```python
from build123d import *

# Parameters (mm, degrees)
BOSS_EXTRUDE1_DEPTH     = 70
SKETCH2_R               = 2.5
CUT_EXTRUDE1_DEPTH      = 81.774377125
CUT_EXTRUDE2_DEPTH      = 81.774377125
CUT_EXTRUDE2_DEPTH_BACK = 81.774377125
SKETCH3_W               = 52
SKETCH3_H               = 57
SKETCH4_R               = 28.5
BOSS_EXTRUDE2_DEPTH     = 52
SKETCH5_R               = 20
BOSS_EXTRUDE3_DEPTH     = 2.5
SKETCH6_R               = 7
BOSS_EXTRUDE4_DEPTH     = 31.5
CUT_EXTRUDE3_DEPTH      = 5


with BuildPart() as part:
    # Sketch1 → Boss-Extrude1 (new body)
    with BuildSketch(Plane.XY):
        Polygon((-28.5, -25.5), (-25.5, -28.5), (25.5, -28.5), (28.5, -25.5), (28.5, 25.5), (25.5, 28.5), (-25.5, 28.5), (-28.5, 25.5), align=None)
    extrude(amount=BOSS_EXTRUDE1_DEPTH)

    # Sketch2 → Cut-Extrude1 (cut, through all)
    with BuildSketch(Plane(origin=(0, 0, 0), x_dir=(-1, 0, 0), z_dir=(0, 0, -1))):
        with Locations((-23.57, 23.57)):
            Circle(SKETCH2_R)
        with Locations((-23.57, -23.57)):
            Circle(SKETCH2_R)
        with Locations((23.57, -23.57)):
            Circle(SKETCH2_R)
        with Locations((23.57, 23.57)):
            Circle(SKETCH2_R)
    extrude(amount=-CUT_EXTRUDE1_DEPTH, mode=Mode.SUBTRACT)

    # Sketch3 → Cut-Extrude2 (cut, two sides: drawn at the far end of the back side and taken through both)
    with BuildSketch(Plane(origin=(0, 0, 0), x_dir=(0, 0, -1), z_dir=(1, 0, 0)).offset(-CUT_EXTRUDE2_DEPTH_BACK)):
        with Locations((-35, 0)):
            Rectangle(SKETCH3_W, SKETCH3_H)
    extrude(amount=CUT_EXTRUDE2_DEPTH + CUT_EXTRUDE2_DEPTH_BACK, mode=Mode.SUBTRACT)


with BuildPart() as cut_extrude2_piece_1:
    # of the separate pieces the step leaves, piece 1, a body of its own (cut_extrude2_pieces)
    add(part.part.solids().sort_by_distance((-28.5, -25.5, 61))[0])



with BuildPart() as cut_extrude2_piece_2:
    # of the separate pieces the step leaves, piece 2, a body of its own (cut_extrude2_pieces)
    add(part.part.solids().sort_by_distance((-28.5, -25.5, 0))[0])


with BuildPart() as cut_extrude2_piece_1_1:
    add(cut_extrude2_piece_1.part)

    add(cut_extrude2_piece_2.part)  # Boss-Extrude2 merges Cut-Extrude2 piece 2
    # Sketch4 → Boss-Extrude2 (add)
    with BuildSketch(Plane.XY.offset(9)):
        with Locations(Location((0, 0, 0), (0, 0, 180))):
            Circle(SKETCH4_R)
    extrude(amount=BOSS_EXTRUDE2_DEPTH)

    # Sketch5 → Boss-Extrude3 (add)
    with BuildSketch(Plane.XY.offset(70)):
        Circle(SKETCH5_R)
    extrude(amount=BOSS_EXTRUDE3_DEPTH)

    # Sketch6 → Boss-Extrude4 (add)
    with BuildSketch(Plane.XY.offset(72.5)):
        Circle(SKETCH6_R)
    extrude(amount=BOSS_EXTRUDE4_DEPTH)

    # Sketch7 → Cut-Extrude3 (cut)
    with BuildSketch(Plane(origin=(0, 9, 0), x_dir=(1, 0, 0), z_dir=(0, 1, 0))):
        with BuildLine():
            Line((-2.5, -98.25), (-2.5, -78.25))
            ThreePointArc((-2.5, -78.25), (0, -75.75), (2.5, -78.25))
            Line((2.5, -78.25), (2.5, -98.25))
            ThreePointArc((2.5, -98.25), (0, -100.75), (-2.5, -98.25))
        make_face()
    extrude(amount=-CUT_EXTRUDE3_DEPTH, mode=Mode.SUBTRACT)


solid = cut_extrude2_piece_1_1.part
```
The listing builds one solid part. Answer for the finished solid, in the listing's coordinates (mm). A direction names the side the tool comes from. Coordinates: 2 decimals unless noted, no trailing zeros. Write each loop counter-clockwise with the first axis right and the second up, starting at its lowest first coordinate (ties: lowest second). Pieces come first, ordered by that corner, then holes. Notation, with made-up numbers: M -32.5,64.5 L 3.5,64.5 A13 cw 3.5,85.5 Z; hole C -6.75,29.5 d4. An arc over 180 degrees is marked long. Use a Markdown table: item, result. Add a question column.
1. Section D-D (x = 15.5) is taken. Give the vertices of the cut face in (y, z).
2. Section A-A (x = -23.57) is taken. Give the vertices of the cut face in (y, z), plus the area to 3 significant figures.
3. Straight lines are drawn through the part: line 1 along Y through (x, z) = (-23.57, 67); line 2 along Y through (x, z) = (23, 65); line 3 along Z through (x, y) = (-25, -16.5). For each, find the intervals that lie inside material, in ascending order. Write a range as [from, to].
4. Which of the six approach directions +Z, -Z, +X, -X, +Y, -Y give full straight-line access (tool end or side, diameter ignored) to faces 1 (the flat face through (-20.6, -22.8, 61)), 2 (the flat face through (21.6, 21.6, 61)), 3 (the cylindrical face through (0.05, 5.52, 100.75))?
5. For a pull along Y with two mould halves and no side action, classify faces 4 (the flat face through (0, -28.5, 65)), 5 (the cylindrical face through (-21.73, 25.26, 4.44)), 6 (the flat face through (-21, 22, 61)) as +Y half, -Y half, draft (parallel to the pull), parting line (faces both ways), or undercut.
6. Section C-C (y = -13) is taken. Give the vertices of the cut face in (x, z), plus the area to 3 significant figures.
7. Given P1, Ø2, axis at y = -5.5, z = 83, coming from the -X side; P2, Ø6.5, axis at x = -23.57, y = -23.57, coming from the +Z side; P3, Ø14, axis at x = -19.5, y = 12.5, coming from the +Z side; P4, Ø3, axis at x = 23.57, y = -23.57, coming from the +Z side, each flat-ended and moving along its own axis, determine where each tip first touches the part or whether it passes through.
Data:
| question | item | result |
|---|---|---|
| 1 | outline | M -28.5,0 L 28.5,0 L 28.5,9 L 23.92,9 L 23.92,61 L 28.5,61 L 28.5,70 L 12.64,70 L 12.64,72.5 L -12.64,72.5 L -12.64,70 L -28.5,70 L -28.5,61 L -23.92,61 L -23.92,9 L -28.5,9 Z |
| 2 | outline | M -28.5,0 L -26.07,0 L -26.07,9 L -28.5,9 Z; M -28.5,61 L -26.07,61 L -26.07,70 L -28.5,70 Z; M -21.07,0 L 21.07,0 L 21.07,9 L 16.02,9 L 16.02,61 L 21.07,61 L 21.07,70 L -21.07,70 L -21.07,61 L -16.02,61 L -16.02,9 L -21.07,9 Z; M 26.07,0 L 28.5,0 L 28.5,9 L 26.07,9 Z; M 26.07,61 L 28.5,61 L 28.5,70 L 26.07,70 Z |
| 2 | area | 2,510 mm2 |
| 3 | line 1 | y = [-28.5, -26.07], [-21.07, 21.07], [26.07, 28.5] |
| 3 | line 2 | y = [-28.5, -26], [-21.14, 21.14], [26, 28.5] |
| 3 | line 3 | z = [0, 9], [61, 70] |
| 4 | face 1 | -X, -Y |
| 4 | face 2 | +X, +Y |
| 4 | face 3 | +Y |
| 5 | face 4 | -Y half |
| 5 | face 5 | undercut |
| 5 | face 6 | draft |
| 6 | outline | M -28.5,0 L 28.5,0 L 28.5,9 L 25.36,9 L 25.36,61 L 28.5,61 L 28.5,70 L 15.2,70 L 15.2,72.5 L -15.2,72.5 L -15.2,70 L -28.5,70 L -28.5,61 L -25.36,61 L -25.36,9 L -28.5,9 Z |
| 6 | area | 3,740 mm2 |
| 7 | P1 | stops at x = -5.36 |
| 7 | P2 | stops at z = 70 |
| 7 | P3 | stops at z = 72.5 |
| 7 | P4 | passes through |
